Autodesk Fusion 360 part; units mm, degrees
sketch "Sketch1" plane through (0, 0, 0) normal (0, 1, 0) x (1, 0, 0)
  line L0 (0, 0) -> (0, -30)
  line L1 (0, -30) -> (50, -30)
  line L2 (50, -30) -> (50, -22.5)
  line L3 (50, -22.5) -> (10, -22.5)
  line L4 (10, -22.5) -> (10, 0)
  line L5 (10, 0) -> (0, 0)
  dimension "d1" = 10
  dimension "d2" = 30
  dimension "d3" = 50
  dimension "d9" = 7.5
extrude "Extrude1" add sketch "Sketch1" along normal blind 40
sketch "Sketch2" plane through (10, 0, 0) normal (1, 0, 0) x (0, 1, 0)
  line L0 (0, 22.5) -> (0, 0)
  line L1 (0, 0) -> (40, 0)
  line L2 (40, 0) -> (40, 22.5)
  line L3 (40, 22.5) -> (0, 22.5)
  line L4 (23.25, 15) -> (23.25, 7.5)
  line L5 (16.75, 7.5) -> (16.75, 15)
  arc A0 (23.25, 15) -> (16.75, 15) centre (20, 15) ccw
  arc A1 (16.75, 7.5) -> (23.25, 7.5) centre (20, 7.5) ccw
  line L6 (0, 0) -> (40, 22.5) construction
  line L7 (20, 15) -> (20, 7.5) construction
  dimension "d6" = 6.5
  dimension "d7" = 7.5
extrude "Extrude2" cut sketch "Sketch2" along normal through all contours L4 L5 A0 A1
fillet "Fillet1" radius 3 2 edges at (0, 20, 30) (50, 20, 30)
Work out the finished part from the listing and answer in its coordinate system (mm). A direction names the side the tool comes from. Give positions to 0.01 mm unless a question says otherwise; leave off trailing zeros. Loops run counter-clockwise (first coordinate to the right, second up) from the corner with the lowest first, then second, coordinate; pieces in that order, holes last. Notation, with made-up numbers: (69, -9) - (114, -9) arc R22 cw to (114, 28) - close; hole circle Ø11 at (24.5, 25). An arc over 180 degrees is marked (long way). Answer in a Markdown table with one row per item.
(1) Section B-B (x = 37.5) is taken. Give the vertices of the cut face in (y, z).
Results list:
| item | result |
|---|---|
| outline | (0, 22.5) - (40, 22.5) - (40, 30) - (0, 30) - close |
(2) A tool of negligible diameter and unlimited length cuts with its end or side. For faces 1 (the face through (10, 20, 11)), 2 (the face through (49.1, 20.28, 29.14)), from which of +Z, -Z, +X, -X, +Y, -Y can it reach the whole face along a straight path? Write none if from no direction.
Results list:
| item | result |
|---|---|
| face 1 | -Z, +X, +Y, -Y |
| face 2 | +Z, +X, +Y, -Y |
(3) Consider L1, parallel to Z at x = 43, y = 16; L2, parallel to X at y = 31, z = 4.5. Determine where each line is inside the solid, lowest interval first. Write a range as [from, to].
Results list:
| item | result |
|---|---|
| L1 | z = [22.5, 30] |
| L2 | x = [0, 10] |
(4) Section C-C (z = 6.75) is taken. Give the vertices of the cut face in (x, y).
Results list:
| item | result |
|---|---|
| outline | (0, 0) - (10, 0) - (10, 40) - (0, 40) - close |
(5) Section A-A (y = 6) is taken. Give the vertices of the cut face in (x, z), and give its area (3 significant figures).
Results list:
| item | result |
|---|---|
| outline | (0, 0) - (10, 0) - (10, 22.5) - (50, 22.5) - (50, 27) arc R3 ccw to (47, 30) - (3, 30) arc R3 ccw to (0, 27) - close |
| area | 596 mm² |
(6) Flat-ended cylindrical pins translate along their axes: pin 1 Ø20 at (x, y) = (39.5, 19) entering from -Z; pin 2 Ø5 at (x, z) = (17.5, 19.5) entering from +Y; pin 3 Ø7 at (y, z) = (20, 12.5) entering from +X. Find the tip coordinate at first contact, or state that the pin passes through.
Results list:
| item | result |
|---|---|
| pin 1 | stops at z = 22.5 |
| pin 2 | passes through |
| pin 3 | stops at x = 10 |
